The model under review builds one solid part; all positions refer to its coordinate system, in mm. Coordinates: 2 decimals unless noted, no trailing zeros. Write each loop counter-clockwise with the first axis right and the second up, starting at its lowest first coordinate (ties: lowest second). Pieces come first, ordered by that corner, then holes. Notation, with made-up numbers: (5.25, 41.5) - (14.25, 41.5) arc R23 ccw to (14.25, 68.5) - close; hole circle Ø5 at (73, -17.5). An arc over 180 degrees is marked (long way). Put each result on its own line as item: value. Start each with the question number.
Item 1: Consider section A-A on z = 0. Give the boundary of the cut face in (x, y).
Item 2: For pin 1 (0.6 mm diameter, centred on y = 0.5, z = 0, fed in from +X); pin 2 (0.7 mm diameter, centred on x = 0, y = 1, fed in from +Z); pin 3 (1 mm diameter, centred on x = -1.5, z = 0.5, fed in from +Y), all flat-tipped, find the tip position at first contact; note any pin that passes through.
Item 3: Consider section C-C on x = -3. Give the boundary of the cut face in (y, z).
Item 4: Mouldability with a two-part tool opening along Y and no side actions: class faces 1 (the face through (-10, 0, 0)), 2 (the face through (-0.846, -2.294, 0.509)), 3 (the face through (-0.6, 0, 0)) as pulls with the +Y half, pulls with the -Y half, needs draft (parallel to the pull), parting line crosses it, or undercut.
Item 5: To check wall thickness, follow L1, parallel to X at y = -0.55, z = -0.2; L2, parallel to X at y = 1.55, z = 0.5; L3, parallel to Y at x = -0.75, z = -0.5. State the ranges of each line that lie inside material, in increasing order. Write a range as [from, to].
Autodesk Inventor part; units mm, degrees
ref_plane "YZ Plane" through (0, 0, 0) normal (1, 0, 0) x (0, 1, 0)
ref_plane "XZ Plane" through (0, 0, 0) normal (0, 1, 0) x (-1, 0, 0)
ref_plane "XY Plane" through (0, 0, 0) normal (0, 0, 1) x (1, 0, 0)
sketch "Sketch1" plane through (0, 0, 0) normal (0, 1, 0) x (-1, 0, 0)
  line L0 (0, 0) -> (1.7, 0)
  line L1 (1.7, 0) -> (1.7, -1.75)
  line L2 (1.1, -2.35) -> (0.6, -2.35)
  line L3 (0, -1.75) -> (0, 0)
  line L4 (1.7, -1.5) -> (10, -1.5)
  line L5 (10, -1.5) -> (10, 0)
  line L6 (10, 0) -> (1.7, 0)
  line L7 (1.7, 0) -> (1.7, -1.5)
  line L8 (1.7, 0) -> (1.7, 2.35)
  line L9 (1.7, 2.35) -> (0, 2.35)
  line L10 (0, 2.35) -> (0, 0)
  line L11 (1.7, 1.5) -> (10, 1.5)
  line L12 (10, 1.5) -> (10, 0)
  arc A0 (1.1, -2.35) -> (1.7, -1.75) centre (1.1, -1.75) ccw
  arc A1 (0, -1.75) -> (0.6, -2.35) centre (0.6, -1.75) ccw
  point P0 (1.7, -2.35)
  point P1 (0, -2.35)
  dimension "d1" = 3
  dimension "d2" = 4.7
  dimension "d3" = 1.7
  dimension "d4" = 10
  dimension "d6" = 0.6
  dimension "d7" = 0.6
revolve "Revolution1" add sketch "Sketch1" angle 360 about axis through (-10, 0, 0) along (1, 0, 0) contours L0 L1 A0 L2 A1 L3 | L6 L5 L4 L1
chamfer "Chamfer1" distance 0.2 angle 45 1 edges at (-10, 0, 1.5)
sketch "Sketch3" plane through (0, 0, 0) normal (0, 1, 0) x (-1, 0, 0)
  line L0 (0.6, 2.35) -> (0.6, -2.35) construction
  line L1 (0, 1.75) -> (0, -1.75)
  line L2 (0, -1.6) -> (1, 0)
  line L3 (1, 0) -> (0, 0)
  line L4 (1, 0) -> (0, 1.6)
  line L5 (0.6, -0.64) -> (0.6, 0.64)
  dimension "d11" = 3.2
  dimension "d12" = 1
  dimension "d18" = 0.6
extrude "Extrusion1" cut sketch "Sketch3" along normal mid plane 0.7 contours L4 L5 L3 L1 | L3 L5 L2 L1
pattern_circular "Circular Pattern1" count 2 over 90 about axis through (-0.85, 0, 0) along (1, 0, 0) of "Extrusion1"
equation "\"d6\" = d7"
properties part number "screw"
Report:
1. outline: (-10, -1.3) - (-9.8, -1.5) - (-1.7, -1.5) - (-1.7, -1.75) arc R0.6 ccw to (-1.1, -2.35) - (-0.6, -2.35) arc R0.6 ccw to (0, -1.75) - (0, -1.6) - (-0.6, -0.64) - (-0.6, 0.64) - (0, 1.6) - (0, 1.75) arc R0.6 ccw to (-0.6, 2.35) - (-1.1, 2.35) arc R0.6 ccw to (-1.7, 1.75) - (-1.7, 1.5) - (-9.8, 1.5) - (-10, 1.3) - close
2. pin 1: x = -0.5
2. pin 2: z = 2.12
2. pin 3: y = 2.34
3. outline: circle Ø3 at (0, 0)
4. face 1: needs draft
4. face 2: parting line crosses it
4. face 3: undercut
5. L1: [-10, -0.6]
5. L2: [-1.7, 0]
5. L3: [-2.3, 2.3]
